Answer from the drawing. Dimensions are ordinates in mm from the lowest x, y and z of the part. A direction names the side the tool comes from. Round coordinates to 2 decimals unless told otherwise and drop trailing zeros. Write each loop counter-clockwise with the first axis right and the second up, starting at its lowest first coordinate (ties: lowest second). Pieces come first, ordered by that corner, then holes. Notation, with made-up numbers: M -0.5,83 L 32.5,83 A23 ccw 32.5,104 Z; hole C 51,5 d4. An arc over 180 degrees is marked long. One line per item, written item: value. Start each with the question number.
(1) Given P1, Ø5, axis at x = 13, y = 46, coming from the +Z side; P2, Ø1.3, axis at x = 0.5, y = 4, coming from the -Z side; P3, Ø1.2, axis at x = 16, y = 25.5, coming from the -Z side, each flat-ended and moving along its own axis, determine where each tip first touches the part or whether it passes through.
(2) Section C-C (z = 2.5) is taken. Determine the outline of the cut face in (x, y).
(3) Section A-A (z = 17.5) is taken. Determine the outline of the cut face in (x, y).
(4) Consider probe 1 along X at (y, z) = (23, 17.5); probe 2 along X at (y, z) = (9, 1); probe 3 along Z at (x, y) = (14.5, 47.5). Determine where each line is inside the solid, lowest interval first.
(5) For a pull along X with two mould halves and no side action, classify the marked faces 4, 5 and 6 as released by +X, released by -X, zero draft, split by the parting line, or undercut.
(6) Section D-D (x = 10.5) is taken. Determine the outline of the cut face in (y, z).
(7) For the marked faces 1, 2 and 3, determine the directions among +Z, -Z, +X, -X, +Y, -Y from which every point of the face is accessible in a straight line to the end or side of a thin tool.
(8) Section B-B (y = 7) is taken. Determine the outline of the cut face in (x, z).
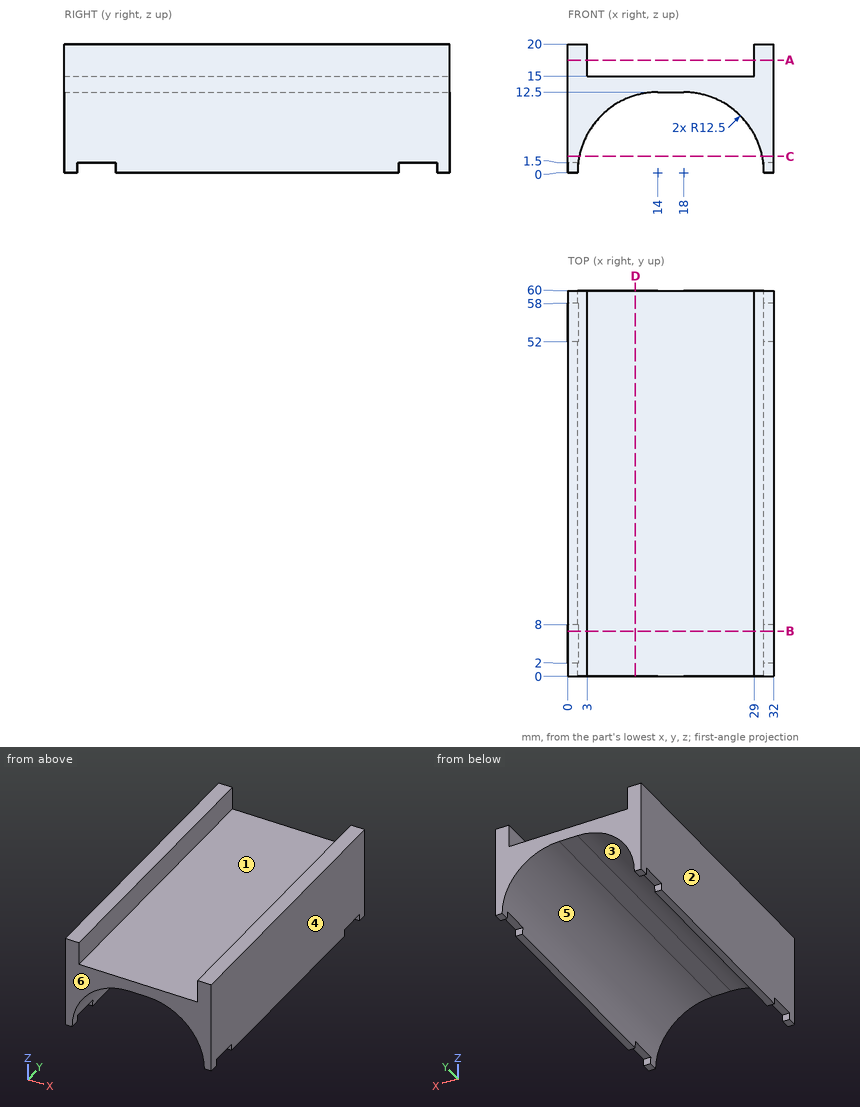
Recorded:
1. P1: stops at z = 15
1. P2: stops at z = 1.5
1. P3: stops at z = 12.5
2. outline: M 0,0 L 1.75,0 L 1.75,60 L 0,60 Z; M 30.25,0 L 32,0 L 32,60 L 30.25,60 Z
3. outline: M 0,0 L 3,0 L 3,60 L 0,60 Z; M 29,0 L 32,0 L 32,60 L 29,60 Z
4. probe 1: x = 0 to 3, 29 to 32
4. probe 2: x = 0 to 1.54, 30.46 to 32
4. probe 3: z = 12.5 to 15
5. face 4: released by +X
5. face 5: undercut
5. face 6: zero draft
6. outline: M 0,12 L 60,12 L 60,15 L 0,15 Z
7. face 1: +Z, +Y, -Y
7. face 2: +Z, -Z, -X, +Y, -Y
7. face 3: -Z, +Y, -Y
8. outline: M 0,1.5 L 1.59,1.5 A12.5 cw 14,12.5 L 18,12.5 A12.5 cw 30.41,1.5 L 32,1.5 L 32,20 L 29,20 L 29,15 L 3,15 L 3,20 L 0,20 Z
